The listing builds one solid part. Answer for the finished solid, in the listing's coordinates (mm). Face numbers are marked on the shaded views. Give positions to 0.01 mm unless a question says otherwise; leave off trailing zeros. Loops run counter-clockwise (first coordinate to the right, second up) from the corner with the lowest first, then second, coordinate; pieces in that order, holes last. Notation, with made-up numbers: (-20.5, -25) -> (19.5, -25) arc R8 cw to (19.5, -11) -> close; hole circle Ø9 at (-28, -8.5). An arc over 180 degrees is marked (long way). One line per question, with ' | ' between items. Start each with the question number.
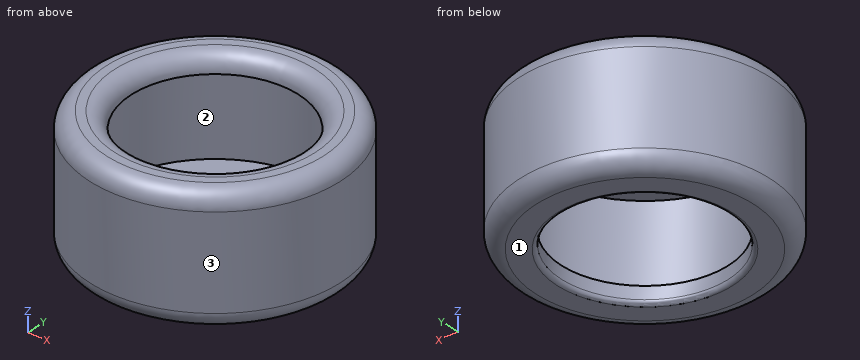
from build123d import *

# Parameters (mm, degrees)
SKETCH1_R           = 15
SKETCH1_R_2         = 10
EXTRUDE_THIN1_DEPTH = 15
FILLET1_R           = 2
FILLET2_R           = 0.5
SHELL5_START        = 2
SHELL5_OUTLINE_R    = 13
SHELL5_OUTLINE_R_2  = 10
SHELL5_DEPTH        = 11


# Read off the part's stored shape, not the designer's step: Shell5
with BuildPart() as part:
    # Sketch1 → Extrude-Thin1 (new body)
    with BuildSketch(Plane.XY):
        Circle(SKETCH1_R)
        Circle(SKETCH1_R_2, mode=Mode.SUBTRACT)
    extrude(amount=EXTRUDE_THIN1_DEPTH)

    # Fillet1
    fillet1_edges = [part.edges().sort_by_distance(p)[0] for p in [
        (-15, 0, 0),
        (-15, 0, 15),
        (-10, 0, 15),
    ]]
    fillet(fillet1_edges, radius=FILLET1_R)

    # Fillet2
    fillet2_edges = [part.edges().sort_by_distance(p)[0] for p in [
        (-10, 0, 0),
    ]]
    fillet(fillet2_edges, radius=FILLET2_R)

    # Shell5 outline → Shell5 (cut)
    with BuildSketch(Plane.XY.offset(SHELL5_START)):
        Circle(SHELL5_OUTLINE_R)
        Circle(SHELL5_OUTLINE_R_2, mode=Mode.SUBTRACT)
    extrude(amount=SHELL5_DEPTH, mode=Mode.SUBTRACT)


solid = part.part
1. The part is cut by section B-B (z = 7). Write down the section's boundary in (x, y).
2. Each of these flat-tipped pins is pushed along its axis until it touches: pin 1 Ø12 at (x, y) = (0, 0) entering from +Z; pin 2 Ø4 at (x, z) = (7.5, 4) entering from -Y; pin 3 Ø2 at (x, z) = (11, 6) entering from -Y; pin 4 Ø6 at (x, z) = (12, 2) entering from +Y. Where does it stop, or does it pass through?
3. The part is cut by section A-A (x = 0). Write down the section's boundary in (y, z).
4. Determine the mould class of the marked faces 1, 2 and 3 for opening direction X: released by +X, released by -X, zero draft, split by the parting line, or undercut.
5. Straight lines are drawn through the part: L1, parallel to Y at x = 0, z = 9.25; L2, parallel to Z at x = -7.25, y = -10.5; L3, parallel to Y at x = -8.25, z = 1.5. For each, find the intervals that lie inside material, in ascending order.
Check sheet entries:
1) outline: circle Ø30 at (0, 0); hole circle Ø26 at (0, 0)
2) pin 1: passes through | pin 2: stops at y = -13.96 | pin 3: stops at y = -11.18 | pin 4: stops at y = 12
3) outline: (-15, 2) arc R2 ccw to (-13, 0) -> (-10.5, 0) arc R0.5 ccw to (-10, 0.5) -> (-10, 2) -> (-13, 2) -> (-13, 13) -> (-10, 13) arc R2 ccw to (-12, 15) -> (-13, 15) arc R2 ccw to (-15, 13) -> close; (10, 0.5) arc R0.5 ccw to (10.5, 0) -> (13, 0) arc R2 ccw to (15, 2) -> (15, 13) arc R2 ccw to (13, 15) -> (12, 15) arc R2 ccw to (10, 13) -> (13, 13) -> (13, 2) -> (10, 2) -> close
4) face 1: zero draft | face 2: undercut | face 3: split by the parting line
5) L1: y = -15 to -13, 13 to 15 | L2: z = 0 to 2, 13 to 15 | L3: y = -12.45 to -5.65, 5.65 to 12.45
